Build history of the part. All positions in model axes, mm. A direction names the side the tool comes from. Give positions to 0.01 mm unless a question says otherwise; leave off trailing zeros. Write each loop counter-clockwise with the first axis right and the second up, starting at its lowest first coordinate (ties: lowest second). Pieces come first, ordered by that corner, then holes. Notation, with made-up numbers: (18.25, -22) - (39.25, -22) arc R13 cw to (39.25, -18) - close; hole circle Ø5 at (30, 23). An arc over 180 degrees is marked (long way). Use one line per item in the form item = value. Start each with the question number.
from build123d import *

# Parameters (mm, degrees)
F1_DEPTH = 120
F2_R     = 2
F3_DEPTH = 95.141


# Not quite as in the source:
# - ends of sketch curves that miss each other by under 0.0002 mm in the source are joined


with BuildPart() as f1:
    # F0 (on Front) → F1 (new body)
    with BuildSketch(Plane.XZ):
        with BuildLine():
            Line((-42.5699986517, 0), (-47.569999482, 0))
            Line((-47.569999482, 0), (-47.569999482, -40))
            ThreePointArc((-47.569999482, -40), (-34.336896153, -72.9223698712), (-2, -87.5279378404))
            Line((-2, -87.5279378404), (-2, -86.0265670688))
            ThreePointArc((-2, -86.0265670688), (0, -86.069999741), (2, -86.0265670688))
            Line((2, -86.0265670688), (2, -87.5279378404))
            ThreePointArc((2, -87.5279378404), (34.336896153, -72.9223698712), (47.569999741, -40))
            Line((47.569999741, -40), (47.570000518, 0))
            Line((47.570000518, 0), (42.570000518, 0))
            Line((42.570000518, 0), (42.570000518, -3.5))
            Line((42.570000518, -3.5), (45.070000518, -3.5))
            Line((45.070000518, -3.5), (45.070000518, -16.9))
            Line((45.070000518, -16.9), (42.570000518, -16.9))
            Line((42.570000518, -16.9), (42.570000518, -40))
            ThreePointArc((42.570000518, -40), (0, -82.5699996948), (-42.5699996948, -40))
            Line((-42.5699996948, -40), (-42.5699986517, -16.9))
            Line((-42.5699986517, -16.9), (-45.070000518, -16.9))
            Line((-45.070000518, -16.9), (-45.070000518, -3.5))
            Line((-45.070000518, -3.5), (-42.5699986517, -3.5))
            Line((-42.5699986517, -3.5), (-42.5699986517, 0))
        make_face()
    extrude(amount=F1_DEPTH)

    # F2 (on face) → F3 (cut, through all)
    with BuildSketch(Plane.YZ.offset(47.570000518)):
        with Locations((-12.29, -10.2)):
            Circle(F2_R)
    extrude(amount=-F3_DEPTH, mode=Mode.SUBTRACT)


solid = f1.part
(1) Which spindle directions (+Z, -Z, +X, -X, +Y, -Y) get a long thin tool onto all of the face, cutting with end or side? Do faces 4 (the flat face through (-45, -59, 0)), 5 (the flat face through (-45.07, -59, -10)), 6 (the cylindrical face through (-0.03, -59.16, -86.07)), 7 (the flat face through (-42.57, -59, -29)). Say none if no direction does.
(2) Cut at D-D, the plane z = -47.5. Give the cut face in (x, y), then the cut area to 3 significant figures.
(3) Cut at C-C, the plane y = -38.5. Give the cut face in (x, z), then the cut area to 3 significant figures.
(4) Two-plate mould, pull along Y, no slides. Class faces 1 (the flat face through (42.57, -59, -2)), 2 (the flat face through (6.8, 0, -82.5)), 3 (the cylindrical face through (46.338, -13.877, -11.417)): +Y half, -Y half, draft (parallel to the pull), parting line (faces both ways), or undercut.
(5) Cut at B-B, the plane z = -10.2. Give the cut face in (x, y).
(6) Pin check, flat tips, straight feed: pin 1 Ø3 at (x, y) = (-44, -80) entering from -Z; pin 2 Ø6 at (x, y) = (19, -81) entering from -Z; pin 3 Ø1.5 at (x, y) = (18, -33) entering from +Z; pin 4 Ø3 at (y, z) = (-12.29, -10.2) entering from +X. Stop position of each tip, or through.
(7) Cut at A-A, the plane y = -12.29. Give the cut face in (x, z), then the cut area to 3 significant figures.
(8) Wall check: line 1 (X direction, y = -109.5, z = -37); line 2 (Y direction, x = 46, z = -10); line 3 (X direction, y = -24.5, z = -12). Give the ranges that are in metal, low to high. Write a range as from..to.
Solution:
q1.face_4 = +Z, +X, -X, +Y, -Y
q1.face_5 = +Y, -Y
q1.face_6 = -Z, +Y, -Y
q1.face_7 = +Z, +Y, -Y
q2.outline = (-46.98, -120) - (-41.9, -120) - (-41.9, 0) - (-46.98, 0) - close; (41.9, -120) - (46.98, -120) - (46.98, 0) - (41.9, 0) - close
q2.area = 1,220 mm2
q3.outline = (-47.57, -40) arc R47.57 ccw to (-2, -87.53) - (-2, -86.03) arc R46.07 ccw to (2, -86.03) - (2, -87.53) arc R47.57 ccw to (47.57, -40) - (47.57, 0) - (42.57, 0) - (42.57, -3.5) - (45.07, -3.5) - (45.07, -16.9) - (42.57, -16.9) - (42.57, -40) arc R42.57 cw to (-42.57, -40) - (-42.57, -16.9) - (-45.07, -16.9) - (-45.07, -3.5) - (-42.57, -3.5) - (-42.57, 0) - (-47.57, 0) - close
q3.area = 1,030 mm2
q4.face_1 = draft
q4.face_2 = +Y half
q4.face_3 = undercut
q5.outline = (-47.57, -120) - (-45.07, -120) - (-45.07, -14.29) - (-47.57, -14.29) - close; (-47.57, -10.29) - (-45.07, -10.29) - (-45.07, 0) - (-47.57, 0) - close; (45.07, -120) - (47.57, -120) - (47.57, -14.29) - (45.07, -14.29) - close; (45.07, -10.29) - (47.57, -10.29) - (47.57, 0) - (45.07, 0) - close
q6.pin_1 = -61.37
q6.pin_2 = -84.8
q6.pin_3 = -78.22
q6.pin_4 = through
q7.outline = (-47.57, -40) arc R47.57 ccw to (-2, -87.53) - (-2, -86.03) arc R46.07 ccw to (2, -86.03) - (2, -87.53) arc R47.57 ccw to (47.57, -40) - (47.57, -12.2) - (45.07, -12.2) - (45.07, -16.9) - (42.57, -16.9) - (42.57, -40) arc R42.57 cw to (-42.57, -40) - (-42.57, -16.9) - (-45.07, -16.9) - (-45.07, -12.2) - (-47.57, -12.2) - close; (-47.57, -8.2) - (-45.07, -8.2) - (-45.07, -3.5) - (-42.57, -3.5) - (-42.57, 0) - (-47.57, 0) - close; (42.57, -3.5) - (45.07, -3.5) - (45.07, -8.2) - (47.57, -8.2) - (47.57, 0) - (42.57, 0) - close
q7.area = 1,010 mm2
q8.line_1 = -47.57..-42.57, 42.57..47.57
q8.line_2 = -120..-14.28, -10.3..0
q8.line_3 = -47.57..-45.07, 45.07..47.57
